Design review of the part built by this model. Coordinates are the model's own, in mm. Face numbers are marked on the shaded views. A direction names the side the tool comes from. Coordinates: 2 decimals unless noted, no trailing zeros. Loops run counter-clockwise (first coordinate to the right, second up) from the corner with the lowest first, then second, coordinate; pieces in that order, holes last. Notation, with made-up numbers: M 74.5,8.25 L 110.5,8.25 A21 cw 110.5,14.25 Z; hole C 42.5,39.5 d4. An arc over 180 degrees is marked long. Put each result on its own line as item: value. Start each with the question number.
(1) Take a section at A-A, the plane x = 16. Give the boundary of the cut face in (y, z).
(2) The part is to be moulded in two halves that separate along X. For the marked faces 3, 4, 5 and 6, say which applies: +X half, -X half, draft (parallel to the pull), parting line (faces both ways), or undercut.
(3) For probe 1 along Y at (x, z) = (0, 1.3); probe 2 along Y at (x, z) = (76.8, -65); probe 3 along X at (y, z) = (66, -25), list the stretches that pass through material, from the lowest coordinate up. Write a range as [from, to].
(4) Take a section at C-C, the plane z = -19. Give the boundary of the cut face in (x, y), then the cut area to 3 significant figures.
(5) Clearance check with flat-ended pins moving along their axes: pin 1 (10 mm diameter, centred on x = -44.5, y = 13.5, fed in from -Z); pin 2 (1.5 mm diameter, centred on x = 76.5, y = 28.5, fed in from +Z); pin 3 (5 mm diameter, centred on x = 0, y = 51, fed in from +Z). State where each tip first meets the part, or that it passes through.
(6) Take a section at B-B, the plane z = -42.5. Give the boundary of the cut face in (x, y).
(7) Take a section at D-D, the plane x = 0. Give the boundary of the cut face in (y, z), then the cut area to 3 significant figures.
(8) For the marked faces 1 and 2, list the 3-axis set-ups (+Z, -Z, +X, -X, +Y, -Y) from which the entire face can be reached by the end or side of a thin tool; tool diameter is ignored.
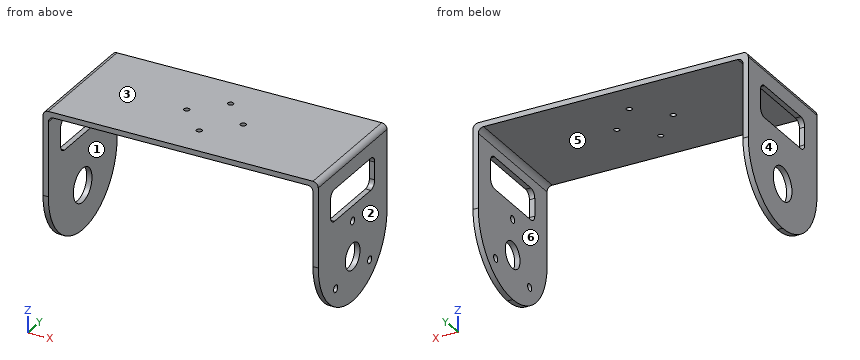
```python
from build123d import *

# Parameters (mm, degrees)
EXTRUDE_1_DEPTH       = 70
FILLET_1_R            = 3
SKETCH_4_R            = 1.55
CUT_EXTRUDE_3_1_DEPTH = 70
SKETCH_13_R           = 2.05
SKETCH_13_R_2         = 7.5
CUT_EXTRUDE_8_DEPTH   = 10
FILLET_6_R            = 35
SKETCH_14_R           = 9.5
CUT_EXTRUDE_9_DEPTH   = 10
SKETCH_15_W           = 18
SKETCH_15_H           = 45
CUT_EXTRUDE_11_DEPTH  = 189.774998345
FILLET_7_R            = 4


with BuildPart() as part:
    # 草图1 → 凸台-拉伸1 (new body)
    with BuildSketch(Plane(origin=(0, 0, 0), x_dir=(1, 0, 0), z_dir=(0, 1, 0))):
        Polygon((-75, 0), (75, 0), (75, 80), (78, 80), (78, -3), (-78, -3), (-78, 80), (-75, 80), align=None)
    extrude(amount=EXTRUDE_1_DEPTH)

    # 圆角1
    fillet_1_edges = [part.edges().sort_by_distance(p)[0] for p in [
        (78, 35, 3),
        (-78, 35, 3),
        (-75, 35, 0),
        (75, 35, 0),
    ]]
    fillet(fillet_1_edges, radius=FILLET_1_R)

    # 草图4 → φ3.1通孔 (cut)
    with BuildSketch(Plane(origin=(0, 0, 0), x_dir=(-1, 0, 0), z_dir=(0, 0, -1))):
        with Locations((0, 51)):
            Circle(SKETCH_4_R)
        with Locations((16, 35)):
            Circle(SKETCH_4_R)
        with Locations((0, 19)):
            Circle(SKETCH_4_R)
        with Locations((-16, 35)):
            Circle(SKETCH_4_R)
    extrude(amount=-CUT_EXTRUDE_3_1_DEPTH, mode=Mode.SUBTRACT)

    # 草图13 → 切除-拉伸8 (cut)
    with BuildSketch(Plane(origin=(78, 0, 0), x_dir=(0, 0, -1), z_dir=(1, 0, 0))):
        with Locations((35, 35)):
            Circle(SKETCH_13_R)
        with Locations((65, 52.320508076)):
            Circle(SKETCH_13_R)
        with Locations((65, 17.679491924)):
            Circle(SKETCH_13_R)
        with Locations((55, 35)):
            Circle(SKETCH_13_R_2)
    extrude(amount=-CUT_EXTRUDE_8_DEPTH, mode=Mode.SUBTRACT)

    # 圆角6
    fillet_6_edges = [part.edges().sort_by_distance(p)[0] for p in [
        (-76.5, 70, -80),
        (-76.5, 0, -80),
        (76.5, 70, -80),
        (76.5, 0, -80),
    ]]
    fillet(fillet_6_edges, radius=FILLET_6_R - 0.0001)  # a hair under: the kernel refuses the full size

    # 草图14 → 切除-拉伸9 (cut)
    with BuildSketch(Plane.ZY.offset(78)):
        with Locations((-55, 35)):
            Circle(SKETCH_14_R)
    extrude(amount=-CUT_EXTRUDE_9_DEPTH, mode=Mode.SUBTRACT)

    # 草图15 → 切除-拉伸11 (cut, through all)
    with BuildSketch(Plane(origin=(78, 0, 0), x_dir=(0, 0, -1), z_dir=(1, 0, 0))):
        with Locations((17.5, 35)):
            Rectangle(SKETCH_15_W, SKETCH_15_H)
    extrude(amount=-CUT_EXTRUDE_11_DEPTH, mode=Mode.SUBTRACT)

    # 圆角7
    fillet_7_edges = [part.edges().sort_by_distance(p)[0] for p in [
        (76.5, 57.5, -26.5),
        (-76.5, 57.5, -26.5),
        (76.5, 12.5, -26.5),
        (-76.5, 12.5, -26.5),
        (76.5, 12.5, -8.5),
        (-76.5, 12.5, -8.5),
        (76.5, 57.5, -8.5),
        (-76.5, 57.5, -8.5),
    ]]
    fillet(fillet_7_edges, radius=FILLET_7_R)


solid = part.part
```
Computed values:
1. outline: M 0,0 L 33.45,0 L 33.45,3 L 0,3 Z; M 36.55,0 L 70,0 L 70,3 L 36.55,3 Z
2. face 3: draft
2. face 4: -X half
2. face 5: undercut
2. face 6: undercut
3. probe 1: y = [0, 17.45], [20.55, 49.45], [52.55, 70]
3. probe 2: y = [6.28, 15.63], [19.73, 50.27], [54.37, 63.72]
3. probe 3: x = [-78, -75], [75, 78]
4. outline: M -78,0 L -75,0 L -75,12.5 L -78,12.5 Z; M -78,57.5 L -75,57.5 L -75,70 L -78,70 Z; M 75,0 L 78,0 L 78,12.5 L 75,12.5 Z; M 75,57.5 L 78,57.5 L 78,70 L 75,70 Z
4. area: 150 mm^2
5. pin 1: stops at z = 0
5. pin 2: stops at z = 2.9
5. pin 3: stops at z = 3
6. outline: M -78,0 L -75,0 L -75,70 L -78,70 Z; M 75,0 L 78,0 L 78,70 L 75,70 Z
7. outline: M 0,0 L 17.45,0 L 17.45,3 L 0,3 Z; M 20.55,0 L 49.45,0 L 49.45,3 L 20.55,3 Z; M 52.55,0 L 70,0 L 70,3 L 52.55,3 Z
7. area: 191 mm^2
8. face 1: -Z, +Y, -Y
8. face 2: +Z, -Z, +X, +Y, -Y
